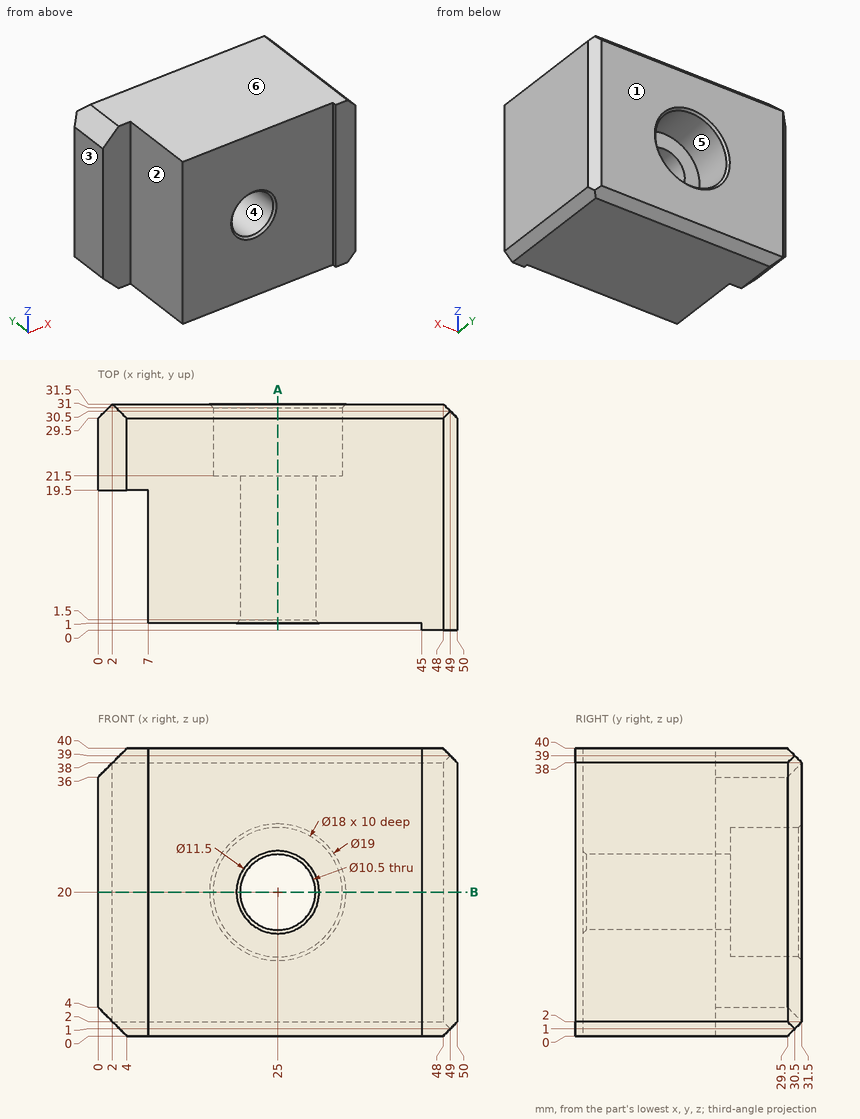
Input: dimensioned drawing with shaded views. Units: mm. Origin: part minimum x, y, z. A direction names the side the tool comes from. Coordinates: 2 decimals unless noted, no trailing zeros. Loops run counter-clockwise (first coordinate to the right, second up) from the corner with the lowest first, then second, coordinate; pieces in that order, holes last. Notation, with made-up numbers: (0, 49) -> (24, 49) arc R7 cw to (24, 62) -> close; hole circle Ø5 at (-25, 54). An arc over 180 degrees is marked (long way). Use a Markdown table: item, result. Add a question column.
(1) Section query A-A, the plane x = 25. Return loops of the section in (y, z), plus the area to 3 significant figures.
(2) Mould query, pull axis X, two halves, no side actions, for the marked faces 3, 4, 5 and 6. Classes: pulls with the +X half, pulls with the -X half, needs draft (parallel to the pull), parting line crosses it, or undercut.
(3) Section query B-B, the plane z = 20. Return loops of the section in (x, y), plus the area to 3 significant figures.
(4) Access query for the marked faces 1 and 2. Directions: +Z, -Z, +X, -X, +Y, -Y. A direction counts if a zero-diameter tool reaches every point of the face in a straight line with its end or side. Return the directions, or none.
(5) Pin query (flat end, axial travel): pin 1 Ø9 at (y, z) = (9, 23.5) entering from -X; pin 2 Ø7.5 at (x, z) = (4, 22.5) entering from -Y; pin 3 Ø14.5 at (x, z) = (25.5, 17) entering from +Y; pin 4 Ø17 at (x, z) = (25, 20) entering from +Y. Return the tip coordinate at first contact, or that it passes through.
(6) Line query: line 1 along Z through (x, y) = (25, 7); line 2 along Z through (x, y) = (25, 26.75); line 3 along X through (y, z) = (10, 20). Output: solid intervals per line, ascending.
Answer:
| question | item | result |
|---|---|---|
| 1 | outline | (1, 0) -> (29.5, 0) -> (31.5, 2) -> (31.5, 10.5) -> (31, 11) -> (21.5, 11) -> (21.5, 14.75) -> (1.5, 14.75) -> (1, 14.25) -> close; (1, 25.75) -> (1.5, 25.25) -> (21.5, 25.25) -> (21.5, 29) -> (31, 29) -> (31.5, 29.5) -> (31.5, 38) -> (29.5, 40) -> (1, 40) -> close |
| 1 | area | 820 mm^2 |
| 2 | face 3 | pulls with the -X half |
| 2 | face 4 | undercut |
| 2 | face 5 | undercut |
| 2 | face 6 | needs draft |
| 3 | outline | (0, 19.5) -> (7, 19.5) -> (7, 1) -> (19.25, 1) -> (19.75, 1.5) -> (19.75, 21.5) -> (16, 21.5) -> (16, 31) -> (15.5, 31.5) -> (2, 31.5) -> (0, 29.5) -> close; (30.25, 1.5) -> (30.75, 1) -> (45, 1) -> (45, 0) -> (50, 0) -> (50, 29.5) -> (48, 31.5) -> (34.5, 31.5) -> (34, 31) -> (34, 21.5) -> (30.25, 21.5) -> close |
| 3 | area | 1,000 mm^2 |
| 4 | face 1 | +Z, -Z, +X, -X, +Y |
| 4 | face 2 | +Z, -Z, -X, -Y |
| 5 | pin 1 | stops at x = 7 |
| 5 | pin 2 | stops at y = 1 |
| 5 | pin 3 | stops at y = 31.5 |
| 5 | pin 4 | stops at y = 21.5 |
| 6 | line 1 | z = 0 to 14.75, 25.25 to 40 |
| 6 | line 2 | z = 0 to 11, 29 to 40 |
| 6 | line 3 | x = 7 to 19.75, 30.25 to 50 |
